Geometry check sheet. Reference: the model listing, model coordinates, mm. A direction names the side the tool comes from. Give positions to 0.01 mm unless a question says otherwise; leave off trailing zeros. Write each loop counter-clockwise with the first axis right and the second up, starting at its lowest first coordinate (ties: lowest second). Pieces come first, ordered by that corner, then holes. Notation, with made-up numbers: (-12.5, 27.25) - (40.5, 27.25) arc R17 cw to (40.5, 32.25) - close; hole circle Ø1 at (75.5, -20). An arc over 180 degrees is marked (long way). Use a Markdown table: item, result.
Autodesk Inventor part; units mm, degrees
ref_plane "YZ Plane" through (0, 0, 0) normal (1, 0, 0) x (0, 1, 0)
ref_plane "XZ Plane" through (0, 0, 0) normal (0, 1, 0) x (-1, 0, 0)
ref_plane "XY Plane" through (0, 0, 0) normal (0, 0, 1) x (1, 0, 0)
sketch "Schizzo1" plane through (0, 0, 0) normal (0, 0, 1) x (1, 0, 0)
  line L0 (100, 75) -> (100, -75)
  line L1 (100, -75) -> (-100, -75)
  line L2 (-100, -75) -> (-100, 75)
  line L3 (-100, 75) -> (100, -75) construction
  line L4 (100, 75) -> (-100, -75) construction
  arc A0 (100, 75) -> (-100, 75) centre (0, 75) ccw
  circle A1 centre (0, 75) radius 67.5
  point P0 (0, 0)
  point P1 (0, 0)
  dimension "d0" = 200
  dimension "d1" = 150
  dimension "d3" = 100
  dimension "d4" = 135
extrude "Piano2" add sketch "Schizzo1" along normal blind 5
sketch "Schizzo2" plane through (-100, -80, -5) normal (0, -1, 0) x (1, 0, 0)
  line L0 (200, 0) -> (0, 0)
  line L1 (0, 0) -> (0, -110)
  line L2 (0, -110) -> (200, -110)
  line L3 (200, -110) -> (200, 0)
edge flange "Flangia1" height 120 angle 90 thickness 5 bend radius 5 thickness toward (0, -1, 0) relief tear relief width 5 relief depth 2.5 edges at (0, -75, 0) wall of the first edge with corners at (100, -80, -5) (-100, -80, -5) (-100, -80, -115) (100, -80, -115)
bend "Piega (Bend)1"
corner "Angolo1"
sketch "Schizzo3" plane through (-100, -79.3301, -117.5) normal (0, -0.8660254, -0.5) x (1, 0, 0)
  line L0 (200, 0) -> (0, 0)
  line L1 (0, 0) -> (0, -87.3205)
  line L2 (0, -87.3205) -> (200, -87.3205)
  line L3 (200, -87.3205) -> (200, 0)
edge flange "Flangia2" height 90 angle 30 thickness 5 bend radius 5 thickness toward (0, -0.8660254, -0.5) relief tear relief width 5 relief depth 2.5 edges at (0, -80, -115) wall of the first edge with corners at (100, -79.3301, -117.5) (-100, -79.3301, -117.5) (-100, -35.6699, -193.1218) (100, -35.6699, -193.1218)
bend "Piega (Bend)2"
corner "Angolo2"
sketch "Schizzo5" plane through (0, 0, 5) normal (0, 0, 1) x (1, 0, 0)
  circle A0 centre (58.3363, 133.3363) radius 6
  circle A1 centre (-58.3363, 133.3363) radius 6
  circle A2 centre (-58.3363, 16.6637) radius 6
  circle A3 centre (58.3363, 16.6637) radius 6
  point P0 (0, 0)
hole "Foro1" at (-58.3363, 133.3363, 5) at (58.3363, 133.3363, 5) at (58.3363, 16.6637, 5) at (-58.3363, 16.6637, 5) direction (0, 0, -1) diameter 12 end through all
sketch "Schizzo6" plane through (-100, -35.6699, -193.1218) normal (0, 0.8660254, 0.5) x (1, 0, 0)
  line L0 (200, 0) -> (0, 0)
  line L1 (100, 0) -> (130, 0)
  line L2 (130, 0) -> (200, -67.3205)
  line L3 (100, 0) -> (70, 0)
  line L4 (0, 0) -> (0, -87.3205)
  line L5 (0, -67.3205) -> (70, 0)
  line L6 (200, -67.3205) -> (200, 19.9941)
  line L7 (200, 19.9941) -> (0, 19.9941)
  line L8 (0, 19.9941) -> (0, -67.3205)
  point P0 (100, -149.4134)
  point P1 (200, -87.3205)
  dimension "d43" = 20
  dimension "d44" = 30
  dimension "d45" = 30
  dimension "d46" = 20
extrude "Taglia1" cut sketch "Schizzo6" against normal blind 5
sketch "Schizzo7" plane through (-30, -31.3397, -195.6218) normal (0, 0, -1) x (-1, 0, 0)
  line L0 (-60, 0) -> (0, 0)
  line L1 (0, 0) -> (0, 24.2265)
  line L2 (0, 24.2265) -> (-60, 24.2265)
  line L3 (-60, 24.2265) -> (-60, 0)
edge flange "Flangia4" height 30 angle 60 thickness 5 bend radius 5 thickness toward (0, 0, -1) relief tear relief width 5 relief depth 2.5 edges at (0, -35.6699, -193.1218) wall of the first edge with corners at (30, -31.3397, -195.6218) (-30, -31.3397, -195.6218) (-30, -7.1132, -195.6218) (30, -7.1132, -195.6218)
bend "Piega (Bend)4"
corner "Angolo4"
fillet "Arrotondamento angolo1" radius 5 2 edges at (30, -7.1132, -198.1218) (-30, -7.1132, -198.1218)
sketch "Schizzo8" plane through (-100, -80, -5) normal (0, 1, 0) x (1, 0, 0)
  circle A0 centre (190, 90) radius 2.5
  point P0 (100, -5)
hole "Foro2" at (90, -80, -95) direction (0, -1, 0) diameter 10 end through all
equation "\"d41\" = Spessore"
equation "\"d47\" = Spessore"
equation "\"d65\" = Spessore"
equation "\"d5\" = Spessore"
equation "\"d6\" = LarghezzaScaricoPiega"
equation "\"d7\" = ProfonditàScaricoPiega"
equation "\"d8\" = ResiduoMinimo"
equation "\"d9\" = RaggioTransizione"
equation "\"d12\" = RaggioPiega"
equation "\"d13\" = DimensioniScaricoAngolo"
equation "\"d14\" = DimensioneGioco"
equation "\"d15\" = Dimensione_raggio_Jacobi"
equation "\"d16\" = LarghezzaScaricoPiega"
equation "\"d17\" = ProfonditàScaricoPiega"
equation "\"d18\" = ResiduoMinimo"
equation "\"d19\" = RaggioTransizione"
equation "\"d22\" = RaggioPiega"
equation "\"d23\" = DimensioniScaricoAngolo"
equation "\"d24\" = DimensioneGioco"
equation "\"d25\" = Dimensione_raggio_Jacobi"
equation "\"d49\" = LarghezzaScaricoPiega"
equation "\"d50\" = ProfonditàScaricoPiega"
equation "\"d51\" = ResiduoMinimo"
equation "\"d52\" = RaggioTransizione"
equation "\"d55\" = RaggioPiega"
equation "\"d56\" = DimensioniScaricoAngolo"
equation "\"d57\" = DimensioneGioco"
equation "\"d58\" = Dimensione_raggio_Jacobi"
equation "\"RaggioPiega\" = Spessore"
equation "\"LarghezzaScaricoPiega\" = Spessore"
equation "\"ProfonditàScaricoPiega\" = 0.5 * Spessore"
equation "\"RaggioTransizione\" = RaggioPiega"
equation "\"Dimensione_raggio_Jacobi\" = RaggioPiega"
equation "\"DimensioneGioco\" = Spessore"
properties part number "Lamiera supporto motore" material "Acciaio inossidabile"
1) Set-up check for faces 1 (the flat face through (-65.5, -54.9, -164.8)), 2 (the flat face through (0, -19, -195.622)): record each of +Z, -Z, +X, -X, +Y, -Y from which the full face is reachable in a straight line by a thin tool's end or side.
Working result:
| item | result |
|---|---|
| face 1 | -Z, -X, +Y |
| face 2 | +X, -X, +Y |
2) Depth check by flat-ended pin: P1, Ø13, axis at x = 90, z = -95, coming from the +Y side; P2, Ø2.5, axis at y = -25, z = -197.5, coming from the +X side; P3, Ø7, axis at x = -58.34, y = 16.66, coming from the -Z side; P4, Ø6, axis at y = -19, z = -196, coming from the -X side. Enter the tip coordinate at first touch or a pass-through.
Working result:
| item | result |
|---|---|
| P1 | stops at y = -80 |
| P2 | stops at x = 30 |
| P3 | passes through |
| P4 | stops at x = -30 |
3) Section check C-C on y = 83.5. Record the boundary of the cut face in (x, z), then the cut area to 3 significant figures.
Working result:
| item | result |
|---|---|
| outline | (-99.64, 0) - (-66.96, 0) - (-66.96, 5) - (-99.64, 5) - close; (66.96, 0) - (99.64, 0) - (99.64, 5) - (66.96, 5) - close |
| area | 327 mm² |
4) Section check B-B on x = 0. Record the boundary of the cut face in (y, z).
Working result:
| item | result |
|---|---|
| outline | (-85, -115) arc R10 ccw to (-83.66, -120) - (-40, -195.62) arc R10 ccw to (-31.34, -200.62) - (-7.11, -200.62) - (-7.11, -195.62) - (-31.34, -195.62) arc R5 cw to (-35.67, -193.12) - (-79.33, -117.5) arc R5 cw to (-80, -115) - (-80, -5) arc R5 cw to (-75, 0) - (7.5, 0) - (7.5, 5) - (-75, 5) arc R10 ccw to (-85, -5) - close; (142.5, 0) - (175, 0) - (175, 5) - (142.5, 5) - close |
5) Section check A-A on z = -95. Record the boundary of the cut face in (x, y).
Working result:
| item | result |
|---|---|
| outline | (-100, -85) - (85, -85) - (85, -80) - (-100, -80) - close; (95, -85) - (100, -85) - (100, -80) - (95, -80) - close |
6) Section check D-D on y = 14.5. Record the boundary of the cut face in (x, z).
Working result:
| item | result |
|---|---|
| outline | (-100, 0) - (-63.93, 0) - (-63.93, 5) - (-100, 5) - close; (-52.74, 0) - (-29.93, 0) - (-29.93, 5) - (-52.74, 5) - close; (29.93, 0) - (52.74, 0) - (52.74, 5) - (29.93, 5) - close; (63.93, 0) - (100, 0) - (100, 5) - (63.93, 5) - close |
7) Material ranges on L1, parallel to Y at x = 83.5, z = -54; L2, parallel to Z at x = 52, y = -39; L3, parallel to Z at x = 90, y = -81.8, recorded low to high. Write a range as from..to.
Working result:
| item | result |
|---|---|
| L1 | y = -85..-80 |
| L2 | z = 0..5 |
| L3 | z = -123.22..-100, -90..2.33 |
8) Mould release check, pull along Y, two halves, no side actions. Record for faces 3 (the cylindrical face through (-56.038, 127.794, 2.465)), 4 (the flat face through (-1.4, -62.657, -146.379)), 5 (the flat face through (100, -40, 2)): pulls with the +Y half, pulls with the -Y half, needs draft (parallel to the pull), parting line crosses it, or undercut.
Working result:
| item | result |
|---|---|
| face 3 | undercut |
| face 4 | pulls with the +Y half |
| face 5 | needs draft |
